Read the model definition and answer for the solid it produces. Units are mm, in the model's axes. A direction names the side the tool comes from. Coordinates: 2 decimals unless noted, no trailing zeros. Order: outer loops, then holes, each group sorted by start corner. A loop starts at its lowest first (then second) coordinate and runs counter-clockwise, first axis right, second up. Notation, with made-up numbers: (50.5, 44.25) - (101.5, 44.25) arc R25 ccw to (101.5, 74.25) - close; hole circle Ø2 at (-33.5, 68.25). An arc over 180 degrees is marked (long way). Use one line per item in the form item = value.
```python
from build123d import *

# Parameters (mm, degrees)
F0_W     = 90.658814
F0_H     = 76.2
F1_DEPTH = 25.4
F2_R     = 5.08
F3_W     = 13.8
F3_H     = 7
F4_DEPTH = 38.608
F5_W     = 13.4
F5_H     = 7
F6_DEPTH = 20.066
F7_R     = 5.926284
F8_DEPTH = 2.032


with BuildPart() as f1:
    # F0 (on Front) → F1 (new body)
    with BuildSketch(Plane.XZ):
        Rectangle(F0_W, F0_H)
    extrude(amount=F1_DEPTH)

    # F2
    f2_edges = [f1.edges().sort_by_distance(p)[0] for p in [
        (0, -25.4, 38.1),
        (0, 0, 38.1),
        (0, 0, -38.1),
        (0, -25.4, -38.1),
    ]]
    fillet(f2_edges, radius=F2_R)

    # F3 (on face) → F4 (cut)
    with BuildSketch(Plane.YZ.offset(45.329407)):
        with Locations((-13.526871, 7.164022)):
            Rectangle(F3_W, F3_H)
    extrude(amount=-F4_DEPTH, mode=Mode.SUBTRACT)

    # F5 (on face) → F6 (cut)
    with BuildSketch(Plane.YZ.offset(45.329407)):
        with Locations((-13.670774, 19.304139)):
            Rectangle(F5_W, F5_H)
    extrude(amount=-F6_DEPTH, mode=Mode.SUBTRACT)

    # F7 (on face) → F8 (join)
    with BuildSketch(Plane.YZ.offset(45.329407)):
        with Locations((-17.124441, -11.080521)):
            Circle(F7_R)
    extrude(amount=F8_DEPTH)


solid = f1.part
```
(1) The mould has two halves that part along Z. Classify faces 3 (the flat face through (35, -20.371, 19)), 4 (the flat face through (-1, 0, 0)), 5 (the cylindrical face through (0.635, -1.528, 36.651)), 6 (the cylindrical face through (0.635, -23.872, -36.651)): +Z half, -Z half, draft (parallel to the pull), parting line (faces both ways), or undercut.
Answer list:
face_3 = undercut
face_4 = draft
face_5 = +Z half
face_6 = -Z half
(2) Given pin 1 Ø2 at (y, z) = (-11.5, 8.5) entering from +X; pin 2 Ø12 at (y, z) = (-21.5, 25) entering from +X, each flat-ended and moving along its own axis, determine where each tip first touches the part or whether it passes through.
Answer list:
pin_1 = 6.72
pin_2 = 45.33
(3) Straight lines are drawn through the part: L1, parallel to Z at x = 37, y = -9; L2, parallel to Z at x = 24, y = -19; L3, parallel to Y at x = 30.5, z = 22. For each, find the intervals that lie inside material, in ascending order.
Answer list:
L1 = -38.1 to 3.66, 10.66 to 15.8, 22.8 to 38.1
L2 = -38.1 to 3.66, 10.66 to 38.1
L3 = -25.4 to -20.37, -6.97 to 0
(4) Which of the six approach directions +Z, -Z, +X, -X, +Y, -Y give full straight-line access (tool end or side, diameter ignored) to faces 1 (the cylindrical face through (0.635, -1.528, -36.651)), 2 (the flat face through (25.263, -14, 19))?
Answer list:
face_1 = -Z, +X, -X, +Y
face_2 = +X
(5) Section D-D, the plane x = 37 is taken. Write down the section's boundary in (y, z).
Answer list:
outline = (-25.4, -33.02) arc R5.08 ccw to (-20.32, -38.1) - (-5.08, -38.1) arc R5.08 ccw to (0, -33.02) - (0, 33.02) arc R5.08 ccw to (-5.08, 38.1) - (-20.32, 38.1) arc R5.08 ccw to (-25.4, 33.02) - close; hole (-20.43, 3.66) - (-6.63, 3.66) - (-6.63, 10.66) - (-20.43, 10.66) - close; hole (-20.37, 15.8) - (-6.97, 15.8) - (-6.97, 22.8) - (-20.37, 22.8) - close
(6) Section B-B, the plane y = -8 is taken. Write down the section's boundary in (x, z).
Answer list:
outline = (-45.33, -38.1) - (45.33, -38.1) - (45.33, 3.66) - (6.72, 3.66) - (6.72, 10.66) - (45.33, 10.66) - (45.33, 15.8) - (25.26, 15.8) - (25.26, 22.8) - (45.33, 22.8) - (45.33, 38.1) - (-45.33, 38.1) - close
(7) Section A-A, the plane x = 19 is taken. Write down the section's boundary in (y, z).
Answer list:
outline = (-25.4, -33.02) arc R5.08 ccw to (-20.32, -38.1) - (-5.08, -38.1) arc R5.08 ccw to (0, -33.02) - (0, 33.02) arc R5.08 ccw to (-5.08, 38.1) - (-20.32, 38.1) arc R5.08 ccw to (-25.4, 33.02) - close; hole (-20.43, 3.66) - (-6.63, 3.66) - (-6.63, 10.66) - (-20.43, 10.66) - close
(8) Section C-C, the plane z = 19 is taken. Write down the section's boundary in (x, y).
Answer list:
outline = (-45.33, -25.4) - (45.33, -25.4) - (45.33, -20.37) - (25.26, -20.37) - (25.26, -6.97) - (45.33, -6.97) - (45.33, 0) - (-45.33, 0) - close
